Part model, mm, in its own coordinate system. A direction names the side the tool comes from. Give positions to 0.01 mm unless a question says otherwise; leave off trailing zeros. Write each loop counter-clockwise with the first axis right and the second up, starting at its lowest first coordinate (ties: lowest second). Pieces come first, ordered by that corner, then holes. Notation, with made-up numbers: M 38.25,13.5 L 57.25,13.5 A26 ccw 57.25,50.5 Z; hole C 53.25,15 d4. An arc over 180 degrees is marked long. Answer as CSV lines item,"result". Start each with the question number.
1) Slice it at D-D, the plane y = 3.75. Give the cut face in (x, z).
2) Mould opens along Z. For faces 1 (the flat face through (-21, 1, 2.901)), 2 (the flat face through (20, 22.38, 13)), 3 (the flat face through (-16, 2.06, 22)) say: pulls with the +Z half, pulls with the -Z half, needs draft (parallel to the pull), parting line crosses it, or undercut.
3) Slice it at C-C, the plane x = 15. Give the cut face in (y, z), plus the area to 3 significant figures.
4) Pin check, flat tips, straight feed: pin 1 Ø5.5 at (y, z) = (7.5, 18) entering from -X; pin 2 Ø6 at (y, z) = (8.5, 15.5) entering from -X; pin 3 Ø8 at (y, z) = (11.5, 37) entering from +X; pin 4 Ø3 at (y, z) = (6, 24) entering from +X. Stop position of each tip, or through.
5) Slice it at A-A, the plane y = 18.5. Give the cut face in (x, z).
6) Slice it at B-B, the plane z = 20.5. Give the cut face in (x, y), plus the area to 3 significant figures.
7) Wall check: line 1 along Z through (x, y) = (14, 14); line 2 along Y through (x, z) = (-22.5, 12.5); line 3 along X through (y, z) = (6.25, 31). Give the ranges that are in metal, low to high. Write a range as from..to.
8) Tool access for faces 4 (the flat face through (20.132, 12.362, 21.712)), 5 (the flat face through (6.756, 20, 21)), 6 (the flat face through (2.166, 1, 5)): list every direction of +Z, -Z, +X, -X, +Y, -Y with a clear straight run to the whole face (end or side of a thin tool).
```python
from build123d import *

# Parameters (mm, degrees)
BOSS_EXTRUDE6_DEPTH  = 2.05994
SKETCH9_W            = 27.13228
SKETCH9_H            = 1.41224
BOSS_EXTRUDE7_DEPTH  = 20.32
SKETCH10_R           = 2.50063
CUT_EXTRUDE3_DEPTH   = 25.4
BOSS_EXTRUDE10_DEPTH = 16.02994


with BuildPart() as part:
    # Sketch8 → Boss-Extrude6 (new body)
    with BuildSketch(Plane(origin=(0, 0, 0), x_dir=(1, 0, 0), z_dir=(0, 1, 0))):
        Polygon((-44.974060072, -2.900891689), (-44.974060072, -40.746891689), (2.165799928, -40.746891689), (2.165799928, -35.808024144), (6.755579928, -31.218244144), (33.887859928, -31.218244144), (33.887859928, -12.429539234), (6.755579928, -12.429539234), (2.165799928, -7.839759234), (2.165799928, -2.900891689), align=None)
    extrude(amount=BOSS_EXTRUDE6_DEPTH)

    # Sketch9 → Boss-Extrude7 (add)
    with BuildSketch(Plane(origin=(0, 2.05994, 0), x_dir=(1, 0, 0), z_dir=(0, 1, 0))):
        with Locations((20.321719928, -13.135659234)):
            Rectangle(SKETCH9_W, SKETCH9_H)
        with Locations((20.321719928, -30.512124144)):
            Rectangle(SKETCH9_W, SKETCH9_H)
    extrude(amount=BOSS_EXTRUDE7_DEPTH)

    # Sketch10 → Cut-Extrude3 (cut)
    with BuildSketch(Plane.XY.offset(31.218244144)):
        with Locations((29.955939928, 17.2847)):
            Circle(SKETCH10_R)
    extrude(amount=-CUT_EXTRUDE3_DEPTH, mode=Mode.SUBTRACT)

    # Sketch14 → Boss-Extrude10 (add)
    with BuildSketch(Plane.XY.offset(13.841779234)):
        Polygon((6.755579928, 22.37994), (33.887859928, 2.05994), (30.568919609, 2.05994), (6.755579928, 19.826826768), align=None)
    extrude(amount=BOSS_EXTRUDE10_DEPTH)


solid = part.part
```
Found:
1,outline,"M 6.76,12.43 L 33.89,12.43 L 33.89,13.84 L 31.63,13.84 L 31.63,29.81 L 33.89,29.81 L 33.89,31.22 L 6.76,31.22 L 6.76,29.81 L 28.3,29.81 L 28.3,13.84 L 6.76,13.84 Z"
2,face 1,"pulls with the -Z half"
2,face 2,"needs draft"
2,face 3,"undercut"
3,outline,"M 0,12.43 L 22.38,12.43 L 22.38,13.84 L 16.21,13.84 L 16.21,29.81 L 22.38,29.81 L 22.38,31.22 L 0,31.22 Z; hole M 2.06,13.84 L 13.68,13.84 L 13.68,29.81 L 2.06,29.81 Z"
3,area,"136 mm²"
4,pin 1,"x = 19.59"
4,pin 2,"x = 6.76"
4,pin 3,"through"
4,pin 4,"x = 30.63"
5,outline,"M 6.76,12.43 L 27.77,12.43 L 27.77,13.84 L 11.94,13.84 L 11.94,29.81 L 27.77,29.81 L 27.77,31.22 L 6.76,31.22 L 6.76,29.81 L 8.53,29.81 L 8.53,13.84 L 6.76,13.84 Z; M 32.14,12.43 L 33.89,12.43 L 33.89,13.84 L 32.14,13.84 Z; M 32.14,29.81 L 33.89,29.81 L 33.89,31.22 L 32.14,31.22 Z"
6,outline,"M -44.97,0 L 33.89,0 L 33.89,2.06 L 6.76,22.38 L 6.76,19.83 L 30.57,2.06 L -44.97,2.06 Z"
6,area,"227 mm²"
7,line 1,"12.43..13.84, 29.81..31.22"
7,line 2,"0..2.06"
7,line 3,"6.76..33.89"
8,face 4,"+X, +Y"
8,face 5,"+Z, -Z, -X, +Y"
8,face 6,"-Z, +X, +Y, -Y"
